Source: CAD feature listing. Evaluate the final solid. Frame: model axes, mm. A direction names the side the tool comes from. Round coordinates to 2 decimals unless told otherwise and drop trailing zeros. Order: outer loops, then holes, each group sorted by start corner. A loop starts at its lowest first (then second) coordinate and runs counter-clockwise, first axis right, second up.
```python
from build123d import *

# Parameters (mm, degrees)
SKETCH1_R           = 3
BOSS_EXTRUDE1_DEPTH = 5


with BuildPart() as part:
    # Sketch1 → Boss-Extrude1 (new body)
    with BuildSketch(Plane(origin=(0, 0, 0), x_dir=(1, 0, 0), z_dir=(0, 1, 0))):
        with BuildLine():
            Line((-25.881865259, -17.986942888), (-11.865528355, -3.931823604))
            ThreePointArc((-11.865528355, -3.931823604), (9.287225619, 8.366447293), (-5.144892732, -11.392105985))
            Line((-5.144892732, -11.392105985), (-18.810797447, -25.0580107))
            ThreePointArc((-18.810797447, -25.0580107), (-25.881865259, -25.0580107), (-25.881865259, -17.986942888))
        make_face()
        with Locations(Location((-22.346331353, -21.522476794, 0), (0, 0, 270))):
            Circle(SKETCH1_R, mode=Mode.SUBTRACT)
        Polygon((0, 10.823922003), (-7.653668647, 7.653668647), (-10.823922003, 0), (-7.653668647, -7.653668647), (0, -10.823922003), (7.653668647, -7.653668647), (10.823922003, 0), (7.653668647, 7.653668647), align=None, mode=Mode.SUBTRACT)
    extrude(amount=BOSS_EXTRUDE1_DEPTH)


solid = part.part
```
1. Access query for faces 1 (the face through (-9, 5, 8)), 2 (the face through (9.261, 2.465, -3.773)). Directions: +Z, -Z, +X, -X, +Y, -Y. A direction counts if a zero-diameter tool reaches every point of the face in a straight line with its end or side. Return the directions, or none.
2. Section C-C on x = 3. Return loops of the section in (y, z).
3. Line query: line 1 along X through (y, z) = (1.8, 22); line 2 along X through (y, z) = (1.55, 23); line 3 along Z through (x, y) = (-22.5, 4). Output: solid intervals per line, ascending.
4. Section A-A on z = -2. Return loops of the section in (x, y).
5. Section B-B on y = 2.3. Return loops of the section in (x, z).
6. Section D-D on z = 13.5. Return loops of the section in (x, y), plus the area to 3 significant figures.
7. Pull-direction query (X, two-part tool) for faces 3 (the face through (-25.803, 2.465, 25.135)), 4 (the face through (-9.261, 2.465, 3.773)), 5 (the face through (-9, 0, 8)); classes: released by +X, released by -X, zero draft, split by the parting line, or undercut.
8. First-contact query: pin 1 (1 mm diameter, centred on y = 4.5, z = 16.5, fed in from +X). Flat tip, straight axial feed; report the tip coordinate or a pass-through.
Result:
1. face 1: +Z, -Z, +X, -X, +Y
1. face 2: +Y, -Y
2. outline: (0, -12.13) - (5, -12.13) - (5, -9.58) - (0, -9.58) - close; (0, 9.58) - (5, 9.58) - (5, 12.13) - (0, 12.13) - close
3. line 1: x = -27.32 to -25.31, -19.38 to -15.75
3. line 2: x = -27.12 to -24.96, -19.74 to -16.75
3. line 3: z = 14.6 to 18.53, 24.52 to 26.52
4. outline: (-12.34, 0) - (-10, 0) - (-10, 5) - (-12.34, 5) - close; (10, 0) - (12.34, 0) - (12.34, 5) - (10, 5) - close
5. outline: (-25.88, 17.99) - (-11.87, 3.93) arc R12.5 ccw (long way) to (-5.14, 11.39) - (-18.81, 25.06) arc R5 ccw to start; hole circle Ø6 at (-22.35, 21.52); hole (-10.82, 0) - (-7.65, -7.65) - (0, -10.82) - (7.65, -7.65) - (10.82, 0) - (7.65, 7.65) - (0, 10.82) - (-7.65, 7.65) - close
6. outline: (-21.41, 0) - (-7.25, 0) - (-7.25, 5) - (-21.41, 5) - close
6. area: 70.8 mm2
7. face 3: split by the parting line
7. face 4: undercut
7. face 5: zero draft
8. pin 1: stops at x = -9.75
